Input: part model. Units: mm. Frame: model coordinates. Round coordinates to 2 decimals unless told otherwise and drop trailing zeros. Order: outer loops, then holes, each group sorted by start corner. A loop starts at its lowest first (then second) coordinate and runs counter-clockwise, first axis right, second up. Notation, with made-up numbers: (-7.5, 88.25) - (35.5, 88.25) arc R21 ccw to (35.5, 119.25) - close; hole circle Ø1 at (39.5, -17). An arc over 180 degrees is marked (long way). One line per item, written item: value. Start each with the question number.
from build123d import *

# Parameters (mm, degrees)
SKETCH1_R           = 1.6
SKETCH1_R_2         = 2.5
BOSS_EXTRUDE1_DEPTH = 3
BOSS_EXTRUDE2_START = -4
SKETCH1_3_R         = 4.75
SKETCH1_3_R_2       = 2.5
BOSS_EXTRUDE2_DEPTH = 4
CUT_EXTRUDE1_DEPTH  = 4
BOSS_EXTRUDE3_START = -3
SKETCH3_R           = 2.5
SKETCH3_R_2         = 1.6
BOSS_EXTRUDE3_DEPTH = 3


with BuildPart() as part:
    # Sketch1 → Boss-Extrude1 (new body)
    with BuildSketch(Plane.XY):
        with BuildLine():
            Line((20.509259259, 2.988776445), (0.410493827, 4.732229371))
            ThreePointArc((0.410493827, 4.732229371), (-4.75, 0), (0.410493827, -4.732229371))
            Line((0.410493827, -4.732229371), (20.509259259, -2.988776445))
            ThreePointArc((20.509259259, -2.988776445), (23.25, 0), (20.509259259, 2.988776445))
        make_face()
        with Locations((16.25, 0)):
            Circle(SKETCH1_R, mode=Mode.SUBTRACT)
        Circle(SKETCH1_R_2, mode=Mode.SUBTRACT)
        with Locations((20.25, 0)):
            Circle(SKETCH1_R, mode=Mode.SUBTRACT)
    extrude(amount=BOSS_EXTRUDE1_DEPTH)

    # Sketch1<3> → Boss-Extrude2 (add)
    with BuildSketch(Plane.XY.offset(BOSS_EXTRUDE2_START)):
        with Locations(Location((0, 0, 0), (0, 0, 85.042328816))):
            Circle(SKETCH1_3_R)
        Circle(SKETCH1_3_R_2, mode=Mode.SUBTRACT)
    extrude(amount=BOSS_EXTRUDE2_DEPTH)

    # Sketch2 → Cut-Extrude1 (cut)
    with BuildSketch(Plane(origin=(0, 0, -4), x_dir=(-1, 0, 0), z_dir=(0, 0, -1))):
        Polygon((-0.133339862, 3), (-0.290232285, 2.483095894), (-0.562101943, 2.9498849), (-0.821593281, 2.888384323), (-0.855050358, 2.349231552), (-1.227240688, 2.740740742), (-1.465554394, 2.6210551), (-1.373772445, 2.088719529), (-1.826218569, 2.383842541), (-2.03050709, 2.212424118), (-1.818434104, 1.715604095), (-2.326744534, 1.898430771), (-2.485994623, 1.684520779), (-2.165063509, 1.25), (-2.701835099, 1.310674107), (-2.807461542, 1.065804489), (-2.394973781, 0.717008082), (-2.931269035, 0.652258663), (-2.977577483, 0.389630403), (-2.495770396, 0.145362072), (-3.002677498, -0.041320215), (-2.987171451, -0.307548759), (-2.462019383, -0.434120444), (-2.91221084, -0.732671509), (-2.835726233, -0.988147888), (-2.295540267, -0.990199415), (-2.664746142, -1.384524292), (-2.53140628, -1.615475708), (-2.005307982, -1.492896479), (-2.27362429, -1.961737012), (-2.090617559, -2.155712815), (-1.606969024, -1.915111108), (-1.759930764, -2.433191983), (-1.537123105, -2.579734886), (-1.121997951, -2.234081601), (-1.151358915, -2.773472944), (-0.900761945, -2.864682781), (-0.576539677, -2.432612176), (-0.480717008, -2.96423526), (-0.215840477, -2.995194886), (0, -2.5), (0.215840477, -2.995194886), (0.480717008, -2.96423526), (0.576539677, -2.432612176), (0.900761945, -2.864682781), (1.151358915, -2.773472944), (1.121997951, -2.234081601), (1.537123105, -2.579734886), (1.759930764, -2.433191983), (1.606969024, -1.915111108), (2.090617559, -2.155712815), (2.27362429, -1.961737012), (2.005307982, -1.492896479), (2.53140628, -1.615475708), (2.664746142, -1.384524292), (2.295540267, -0.990199415), (2.835726233, -0.988147888), (2.91221084, -0.732671509), (2.462019383, -0.434120444), (2.987171451, -0.307548759), (3.002677498, -0.041320215), (2.495770396, 0.145362072), (2.977577483, 0.389630403), (2.931269035, 0.652258663), (2.394973781, 0.717008082), (2.807461542, 1.065804489), (2.701835099, 1.310674107), (2.165063509, 1.25), (2.485994623, 1.684520779), (2.326744534, 1.898430771), (1.818434104, 1.715604095), (2.03050709, 2.212424118), (1.826218569, 2.383842541), (1.373772445, 2.088719529), (1.465554394, 2.6210551), (1.227240688, 2.740740742), (0.855050358, 2.349231552), (0.821593281, 2.888384323), (0.562101943, 2.9498849), (0.290232285, 2.483095894), (0.133339862, 3), align=None)
    extrude(amount=-CUT_EXTRUDE1_DEPTH, mode=Mode.SUBTRACT)

    # Sketch3 → Boss-Extrude3 (add)
    with BuildSketch(Plane.XY.offset(3).offset(BOSS_EXTRUDE3_START)):
        Circle(SKETCH3_R)
        Circle(SKETCH3_R_2, mode=Mode.SUBTRACT)
    extrude(amount=BOSS_EXTRUDE3_DEPTH)


solid = part.part
1. Section A-A (z = 2.75). Return the cut outline in (x, y).
2. Section B-B (x = 20.25). Return the cut outline in (y, z).
3. Section D-D (x = 7.5). Return the cut outline in (y, z).
4. Pin query (flat end, axial travel): pin 1 (1.8 mm diameter, centred on x = -1, y = 1, fed in from -Z); pin 2 (1.5 mm diameter, centred on x = 3.5, z = 0, fed in from +Y). Return the tip coordinate at first contact, or that it passes through.
5. Line query: line 1 (X direction, y = 0.25, z = -1); line 2 (X direction, y = -0.5, z = -1.5); line 3 (Z direction, x = 21.5, y = 2). Output: solid intervals per line, ascending. Write a range as from..to.
6. Pull-direction query (X, two-part tool) for faces 1 (the face through (14.65, 0.07, 1.48)), 2 (the face through (10.6, 3.85, 1.48)), 3 (the face through (-1.27, -0.97, 1.48)), 4 (the face through (9, 0, 3)); classes: released by +X, released by -X, zero draft, split by the parting line, or undercut.
7. Section C-C (x = 16.25). Return the cut outline in (y, z).
Solved:
1. outline: (0.41, -4.73) - (20.51, -2.99) arc R3 ccw to (20.51, 2.99) - (0.41, 4.73) arc R4.75 ccw (long way) to start; hole circle Ø3.2 at (0, 0); hole circle Ø3.2 at (16.25, 0); hole circle Ø3.2 at (20.25, 0)
2. outline: (-3.01, 0) - (-1.6, 0) - (-1.6, 3) - (-3.01, 3) - close; (1.6, 0) - (3.01, 0) - (3.01, 3) - (1.6, 3) - close
3. outline: (-4.12, 0) - (4.12, 0) - (4.12, 3) - (-4.12, 3) - close
4. pin 1: stops at z = 0
4. pin 2: stops at y = 4.53
5. line 1: x = -4.74..-2.7, 2.7..4.74
5. line 2: x = -4.72..-2.56, 2.56..4.72
5. line 3: z = 0..3
6. face 1: undercut
6. face 2: released by +X
6. face 3: undercut
6. face 4: zero draft
7. outline: (-3.36, 0) - (-1.6, 0) - (-1.6, 3) - (-3.36, 3) - close; (1.6, 0) - (3.36, 0) - (3.36, 3) - (1.6, 3) - close
